Could you check a few things on this model? Use its own coordinates, in mm. A direction names the side the tool comes from. Give positions to 0.01 mm unless a question says otherwise; leave off trailing zeros. Order: outer loops, then holes, each group sorted by start corner. A loop starts at its lowest first (then second) coordinate and runs counter-clockwise, first axis right, second up. Notation, with made-up numbers: M 72,7 L 125,7 A14 ccw 125,33 Z; hole C -34.5,85.25 d10. An arc over 180 degrees is marked long. Return JSON: item names as keys, results as strings. Group by question number.
```python
from build123d import *

# Parameters (mm, degrees)
SKETCH1_R           = 11.25
SKETCH1_R_2         = 1.75
BOSS_EXTRUDE1_DEPTH = 5
BOSS_EXTRUDE2_DEPTH = 46
BOSS_EXTRUDE3_DEPTH = 20
CUT_EXTRUDE1_DEPTH  = 1
CUT_EXTRUDE2_DEPTH  = 65.090268372
CUT_EXTRUDE3_REACH  = 71.748
SKETCH6_R           = 2.7
SKETCH6_R_2         = 3.2
CUT_EXTRUDE4_REACH  = 70.949
SKETCH7_R           = 5.2
SKETCH7_R_2         = 3.2
SKETCH8_R           = 3.05
CUT_EXTRUDE5_DEPTH  = 2
FILLET1_R           = 2.5
FILLET2_R           = 5
FILLET3_R           = 0.5


with BuildPart() as part:
    # Sketch1 → Boss-Extrude1 (new body)
    with BuildSketch(Plane.XY):
        Polygon((-13.5, 34.75), (-28, 20.25), (-28, -7.25), (-0.5, -7.25), (-0.5, -34.75), (7, -34.75), (28, -13.75), (28, 29.75), (23, 34.75), align=None)
        with Locations((7, 13.75)):
            Circle(SKETCH1_R, mode=Mode.SUBTRACT)
        with Locations((-8.5, 29.25)):
            Circle(SKETCH1_R_2, mode=Mode.SUBTRACT)
        with Locations(Location((22.5, 29.25, 0), (0, 0, 180))):
            Circle(SKETCH1_R_2, mode=Mode.SUBTRACT)
        with Locations((22.5, -1.75)):
            Circle(SKETCH1_R_2, mode=Mode.SUBTRACT)
    extrude(amount=BOSS_EXTRUDE1_DEPTH)

    # Sketch2 → Boss-Extrude2 (add)
    with BuildSketch(Plane.XY.offset(5)):
        Polygon((-28, -7.25), (-0.5, -7.25), (-0.5, -34.75), (4.5, -34.75), (4.5, -2.25), (-28, -2.25), align=None)
    extrude(amount=BOSS_EXTRUDE2_DEPTH)

    # Sketch3 → Boss-Extrude3 (add)
    with BuildSketch(Plane(origin=(0, -2.25, 0), x_dir=(1, 0, 0), z_dir=(0, 1, 0))):
        with BuildLine():
            Line((-28, -5), (-28, -17.6))
            Line((-28, -17.6), (-19.6, -26))
            Line((-19.6, -26), (-11.4, -26))
            Line((-11.4, -26), (-4.2, -18.8))
            Line((-4.2, -18.8), (-4.2, -5))
            Line((-4.2, -5), (-18.5, -5))
            Line((-18.5, -5), (-18.5, -11.752647884))
            ThreePointArc((-18.5, -11.752647884), (-11.96959369, -19.81788309), (-19.5, -12.677350455))
            Line((-19.5, -12.677350455), (-19.5, -5))
            Line((-19.5, -5), (-28, -5))
        make_face()
    extrude(amount=BOSS_EXTRUDE3_DEPTH)

    # Sketch4 → Cut-Extrude1 (cut)
    with BuildSketch(Plane(origin=(0, -2.25, 0), x_dir=(1, 0, 0), z_dir=(0, 1, 0))):
        with BuildLine():
            Line((-28, -17.6), (-28, 0))
            Line((-28, 0), (-18.5, 0))
            Line((-18.5, 0), (-18.5, -11.752647884))
            ThreePointArc((-18.5, -11.752647884), (-20.681128714, -15.55738815), (-19.176955262, -19.676955262))
            Line((-19.176955262, -19.676955262), (-22.55, -23.05))
            Line((-22.55, -23.05), (-28, -17.6))
        make_face()
    extrude(amount=CUT_EXTRUDE1_DEPTH, mode=Mode.SUBTRACT)

    # Sketch5 → Cut-Extrude2 (cut, through all)
    with BuildSketch(Plane.XY.offset(5)):
        Polygon((-19.5, 17.75), (-28, 17.75), (-28, 18.75), (-18.5, 18.75), (-18.5, -1.25), (-19.5, -1.25), align=None)
    extrude(amount=-CUT_EXTRUDE2_DEPTH, mode=Mode.SUBTRACT)

    # Sketch6 → Cut-Extrude3 (cut, up to next)
    with BuildSketch(Plane(origin=(4.5, 0, 0), x_dir=(0, 0, -1), z_dir=(1, 0, 0)), mode=Mode.PRIVATE) as cut_extrude3_sk1:
        with Locations((-16, -22.25)):
            Circle(SKETCH6_R)
    cut_extrude3_tool1 = extrude(cut_extrude3_sk1.sketch, amount=-CUT_EXTRUDE3_REACH, mode=Mode.PRIVATE) & part.part
    # Sketch6 → Cut-Extrude3 (cut, up to next)
    with BuildSketch(Plane(origin=(4.5, 0, 0), x_dir=(0, 0, -1), z_dir=(1, 0, 0)), mode=Mode.PRIVATE) as cut_extrude3_sk2:
        with Locations((-37.5, -22.25)):
            Circle(SKETCH6_R_2)
    cut_extrude3_tool2 = extrude(cut_extrude3_sk2.sketch, amount=-CUT_EXTRUDE3_REACH, mode=Mode.PRIVATE) & part.part
    add(cut_extrude3_tool1.solids().sort_by_distance((4.5, -22.25, 16))[0], mode=Mode.SUBTRACT)
    add(cut_extrude3_tool2.solids().sort_by_distance((4.5, -22.25, 37.5))[0], mode=Mode.SUBTRACT)

    # Sketch7 → Cut-Extrude4 (cut, up to next)
    with BuildSketch(Plane(origin=(0, -2.25, 0), x_dir=(1, 0, 0), z_dir=(0, 1, 0)), mode=Mode.PRIVATE) as cut_extrude4_sk1:
        with Locations(Location((-15.5, -16, 0), (0, 0, 125.234417985))):
            Circle(SKETCH7_R)
    cut_extrude4_tool1 = extrude(cut_extrude4_sk1.sketch, amount=-CUT_EXTRUDE4_REACH, mode=Mode.PRIVATE) & part.part
    # Sketch7 → Cut-Extrude4 (cut, up to next)
    with BuildSketch(Plane(origin=(0, -2.25, 0), x_dir=(1, 0, 0), z_dir=(0, 1, 0)), mode=Mode.PRIVATE) as cut_extrude4_sk2:
        with Locations(Location((-15.5, -37.5, 0), (0, 0, 270))):
            Circle(SKETCH7_R_2)
    cut_extrude4_tool2 = extrude(cut_extrude4_sk2.sketch, amount=-CUT_EXTRUDE4_REACH, mode=Mode.PRIVATE) & part.part
    add(cut_extrude4_tool1.solids().sort_by_distance((-15.5, -2.25, 16))[0], mode=Mode.SUBTRACT)
    add(cut_extrude4_tool2.solids().sort_by_distance((-15.5, -2.25, 37.5))[0], mode=Mode.SUBTRACT)

    # Sketch8 → Cut-Extrude5 (cut)
    with BuildSketch(Plane.XY.offset(5)):
        with Locations((-8.5, 29.25)):
            Circle(SKETCH8_R)
    extrude(amount=-CUT_EXTRUDE5_DEPTH, mode=Mode.SUBTRACT)

    # Sketch9 → Cut-Revolve1 (revolve, cut)
    with BuildSketch(Plane(origin=(0, 7.75, 0), x_dir=(1, 0, 0), z_dir=(0, 1, 0)), mode=Mode.PRIVATE) as cut_revolve1_sk:
        Polygon((-4.2, -9), (-4.2, -6), (-7.2, -6), (-7.2, -7.25), (-23, -7.25), (-23, -6.65), (-27, -6.65), (-27, -6.5), (-28, -6.5), (-28, -9), align=None)
    revolve(cut_revolve1_sk.sketch.rotate(Axis((-38.14027768, 7.75, 9), (1, 0, 0)), 180), axis=Axis((-38.14027768, 7.75, 9), (1, 0, 0)), mode=Mode.SUBTRACT)

    # Fillet1
    fillet1_edges = [part.edges().sort_by_distance(p)[0] for p in [
        (4.5, -2.25, 28),
        (-28, 20.25, 2.5),
        (7, -34.75, 2.5),
        (28, -13.75, 2.5),
        (28, 29.75, 2.5),
        (23, 34.75, 2.5),
        (-13.5, 34.75, 2.5),
    ]]
    fillet(fillet1_edges, radius=FILLET1_R)

    # Fillet2
    fillet2_edges = [part.edges().sort_by_distance(p)[0] for p in [
        (-28, 8.25, 17.6),
        (-4.2, 7.75, 18.8),
    ]]
    fillet(fillet2_edges, radius=FILLET2_R)

    # Fillet3
    # the kernel refuses this fillet: 0.5 mm, written as the material it takes off along each edge
    with BuildSketch(Plane(origin=(-28, -1.25, 15.528932188), x_dir=(1, 0, 0), z_dir=(0, 0, -1)), Plane(origin=(-28, 17.75, -1.25), x_dir=(1, 0, 0), z_dir=(0, 0, 1))) as fillet3_piece_1:
        with BuildLine():
            CenterArc((FILLET3_R, -FILLET3_R), FILLET3_R, 90, 90)
            Line((0, -FILLET3_R), (0, 0))
            Line((0, 0), (FILLET3_R, 0))
        make_face()
    extrude(amount=16.778932188, mode=Mode.SUBTRACT)
    with BuildSketch(Plane(origin=(-28, 18.75, 6.272209074), x_dir=(0.0007754462768724465, 0.9999996993414906, 0), z_dir=(0, 0, -1))) as fillet3_piece_2:
        with BuildLine():
            CenterArc((0.500387818, 0.499927816), FILLET3_R, 179.955570197, 91.018024984)
            Line((0.000387968, 0.500315539), (-0.049612017, 0.500354311))
            Line((-0.049612017, 0.500354311), (-0.049999985, 3.8772e-05))
            Line((-0.049999985, 3.8772e-05), (-3.8772e-05, -0.049999985))
            ThreePointArc((-3.8772e-05, -0.049999985), (0.464427182, -0.050360153), (0.509733211, -0.049992782))
            Line((0.509733211, -0.049992782), (0.508883629, 0))
        make_face()
    extrude(amount=7.544418147, mode=Mode.SUBTRACT)
    with BuildSketch(Plane(origin=(-28, -7.25, -1.25), x_dir=(0, 1, 0), z_dir=(0, 0, 1))) as fillet3_piece_3:
        with BuildLine():
            CenterArc((FILLET3_R, -FILLET3_R), FILLET3_R, 90, 90)
            Line((0, -FILLET3_R), (0, 0))
            Line((0, 0), (FILLET3_R, 0))
        make_face()
    extrude(amount=53.5, mode=Mode.SUBTRACT)
    with BuildSketch(Plane(origin=(-26.535533906, 17.75, 19.064466094), x_dir=(0, -1, 0), z_dir=(0.707106781186549, 0, 0.707106781186546))) as fillet3_piece_4:
        with BuildLine():
            CenterArc((FILLET3_R, FILLET3_R), FILLET3_R, 180, 90)
            Line((0, FILLET3_R), (0, 0))
            Line((0, 0), (FILLET3_R, 0))
        make_face()
    extrude(amount=11.058326112, mode=Mode.SUBTRACT)
    with BuildSketch(Plane(origin=(-22.55, -1.25, 23.05), x_dir=(0, 1, 0), z_dir=(-0.7071067811865489, 0, -0.7071067811865461))) as fillet3_piece_5:
        with BuildLine():
            CenterArc((FILLET3_R, FILLET3_R), FILLET3_R, 180, 90)
            Line((0, FILLET3_R), (0, 0))
            Line((0, 0), (FILLET3_R, 0))
        make_face()
    extrude(amount=5.636396103, mode=Mode.SUBTRACT)
    with BuildSketch(Plane(origin=(-23, -1.25, 15.528932188), x_dir=(-0.7071067811865456, 0, 0.7071067811865495), z_dir=(0.7071067811865495, 0, 0.7071067811865456))) as fillet3_piece_6:
        with BuildLine():
            CenterArc((5 - FILLET3_R, -FILLET3_R), FILLET3_R, 0, 90)
            Line((5, -FILLET3_R), (5, 0))
            Line((5, 0), (5 - FILLET3_R, 0))
        make_face()
    revolve(axis=Axis((-23, -1.25, 15.528932188), (0, -1, 0)), revolution_arc=45, mode=Mode.SUBTRACT)
    with BuildSketch(Plane(origin=(-4.2, 17.75, 16.728932188), x_dir=(0, -1, 0), z_dir=(0, 0, -1))) as fillet3_piece_7:
        with BuildLine():
            CenterArc((FILLET3_R, FILLET3_R), FILLET3_R, 180, 90)
            Line((0, FILLET3_R), (0, 0))
            Line((0, 0), (FILLET3_R, 0))
        make_face()
    extrude(amount=11.728932188, mode=Mode.SUBTRACT)
    with BuildSketch(Plane(origin=(-9.2, 17.75, 16.728932188), x_dir=(1, 0, 0), z_dir=(0, 0, -1))) as fillet3_piece_8:
        with BuildLine():
            CenterArc((5 - FILLET3_R, FILLET3_R), FILLET3_R, 270, 90)
            Line((5 - FILLET3_R, 0), (5, 0))
            Line((5, 0), (5, FILLET3_R))
        make_face()
    revolve(axis=Axis((-9.2, 17.75, 16.728932188), (0, -1, 0)), revolution_arc=45, mode=Mode.SUBTRACT)
    with BuildSketch(Plane(origin=(-23, 17.75, 15.528932188), x_dir=(-0.7071067811865456, 0, 0.7071067811865495), z_dir=(0.7071067811865495, 0, 0.7071067811865456))) as fillet3_piece_9:
        with BuildLine():
            CenterArc((5 - FILLET3_R, FILLET3_R), FILLET3_R, 270, 90)
            Line((5, FILLET3_R), (5, 0))
            Line((5, 0), (5 - FILLET3_R, 0))
        make_face()
    revolve(axis=Axis((-23, 17.75, 15.528932188), (0, -1, 0)), revolution_arc=45, mode=Mode.SUBTRACT)
    with BuildSketch(Plane(origin=(-28, -2.25, 52.25), x_dir=(1, 0, 0), z_dir=(0, 0, -1))) as fillet3_piece_10:
        with BuildLine():
            CenterArc((FILLET3_R, FILLET3_R), FILLET3_R, 180, 90)
            Line((0, FILLET3_R), (0, 0))
            Line((0, 0), (FILLET3_R, 0))
        make_face()
    extrude(amount=53.5, mode=Mode.SUBTRACT)
    with BuildSketch(Plane(origin=(-18.5, -2.25, 11.752647884), x_dir=(0, 0, -1), z_dir=(0, 1, 0))) as fillet3_piece_11:
        with BuildLine():
            CenterArc((0.875147274, -0.5), FILLET3_R, 90, 116.014366)
            ThreePointArc((0.425805222, -0.719298246), (0.22737913, -0.351079413), (0, 0))
            Line((0, 0), (0.875147274, 0))
        make_face()
    extrude(amount=22.187868184, mode=Mode.SUBTRACT)
    with BuildSketch(Plane(origin=(-12.283883476, 17.75, 26.883883476), x_dir=(0, -1, 0), z_dir=(0.7071067811865485, 0, -0.7071067811865467))) as fillet3_piece_12:
        with BuildLine():
            CenterArc((FILLET3_R, FILLET3_R), FILLET3_R, 180, 90)
            Line((0, FILLET3_R), (0, 0))
            Line((0, 0), (FILLET3_R, 0))
        make_face()
    extrude(amount=9.361269837, mode=Mode.SUBTRACT)
    with BuildSketch(Plane(origin=(-18.5, 17.75, 5), x_dir=(0, -1, 0), z_dir=(0, 0, 1))) as fillet3_piece_13:
        with BuildLine():
            CenterArc((FILLET3_R, FILLET3_R), FILLET3_R, 180, 90)
            Line((0, FILLET3_R), (0, 0))
            Line((0, 0), (FILLET3_R, 0))
        make_face()
    extrude(amount=8.002647884, mode=Mode.SUBTRACT)
    with BuildSketch(Plane(origin=(-19.5, 17.75, 13.927350455), x_dir=(-1, 0, 0), z_dir=(0, 0, -1))) as fillet3_piece_14:
        with BuildLine():
            CenterArc((FILLET3_R, -FILLET3_R), FILLET3_R, 90, 90)
            Line((0, -FILLET3_R), (0, 0))
            Line((0, 0), (FILLET3_R, 0))
        make_face()
    extrude(amount=15.177350455, mode=Mode.SUBTRACT)
    with BuildSketch(Plane(origin=(-19.5, -1.25, 13.927350455), x_dir=(-1, 0, 0), z_dir=(0, 0, -1))) as fillet3_piece_15:
        with BuildLine():
            CenterArc((FILLET3_R, FILLET3_R), FILLET3_R, 180, 90)
            Line((0, FILLET3_R), (0, 0))
            Line((0, 0), (FILLET3_R, 0))
        make_face()
    extrude(amount=15.177350455, mode=Mode.SUBTRACT)


with BuildPart() as body_2:
    # Mirror1: mirrored copy
    add(part.part.mirror(Plane(origin=(0, 0, 0), x_dir=(0, 0, 1), z_dir=(1, 0, 0))))


solid = body_2.part
```
1. Imagine slicing it at A-A, the plane y = 13.75. Please give me the cut outline in (x, z).
2. Imagine slicing it at B-B, the plane x = 3. Please give me the cut outline in (y, z), plus the area to 3 significant figures.
3. If we mould it in two halves opening along X, with no side actions, what happens to faces 1 (the flat face through (-28, 8, 2)), 2 (the flat face through (-5, 34.75, 2)), 3 (the cylindrical face through (-12.19, 3.77, 2.46))? For each: pulls with the +X half, pulls with the -X half, needs draft (parallel to the pull), parting line crosses it, or undercut.
4. Imagine slicing it at D-D, the plane z = 37. Please give me the cut outline in (x, y).
5. I need wall thicknesses on L1, parallel to Z at x = 13, y = 8.5; L2, parallel to Z at x = -1.5, y = -24.5; L3, parallel to X at y = 29.25, z = 1.55. Which ranges of each line are inside material? Lowest first, please. Write a range as from..to.
6. For pin 1 (2 mm diameter, centred on x = -5, z = 45, fed in from +Y); pin 2 (9 mm diameter, centred on x = 6, z = 21, fed in from +Y); pin 3 (1.5 mm diameter, centred on x = 23.5, z = 2.5, fed in from -Y); pin 4 (5 mm diameter, centred on y = -22.25, z = 16, fed in from -X), each with a flat end and sliding along its axis, tell me the tip position at first contact or that it passes through.
7. Which directions (+Z, -Z, +X, -X, +Y, -Y) give clear straight access to the entire face, cutting with the end or side of a thin tool? Please do faces 4 (the flat face through (23, 8, 11)), 5 (the flat face through (7.2, 8, 11)), 6 (the flat face through (23, 18.75, 3)).
8. Imagine slicing it at C-C, the plane y = -22.25. Please give me the cut outline in (x, z), plus the area to 3 significant figures.
Values:
{
 "1": {"outline": "M -28,0 L -18.25,0 L -18.25,5 L -28,5 Z; M 4.2,5 L 4.25,5 L 4.25,0 L 18.5,0 L 18.5,10.88 A0.5 ccw 17.78,11.33 A5.2 cw long 19.5,12.68 L 19.5,0 L 28,0 L 28,15.53 A5 ccw 26.54,19.06 L 19.6,26 L 11.4,26 L 5.66,20.26 A5 ccw 4.2,16.73 Z"},
 "2": {"outline": "M -7.25,0 L 8.6,0 L 8.6,5 L -2.25,5 L -2.25,51 L -7.25,51 Z; M 18.9,0 L 34.75,0 L 34.75,5 L 18.9,5 Z", "area": "388 mm²"},
 "3": {"face 1": "pulls with the -X half", "face 2": "needs draft", "face 3": "undercut"},
 "4": {"outline": "M -4.5,-34.75 L 0.5,-34.75 L 0.5,-25.41 L -4.5,-25.41 Z; M -4.5,-19.09 L 0.5,-19.09 L 0.5,-7.25 L 12.34,-7.25 L 12.34,-2.25 L -2,-2.25 A2.5 ccw -4.5,-4.75 Z; M 18.66,-7.25 L 27.5,-7.25 A0.5 ccw 28,-6.75 L 28,-2.75 A0.5 ccw 27.5,-2.25 L 18.66,-2.25 Z"},
 "5": {"L1": "z = 0..7.42, 10.58..11.44, 20.56..26", "L2": "z = 0..14.51, 17.49..35.22, 39.78..51", "L3": "x = -27.94..-24.25, -20.75..6.75, 10.25..19"},
 "6": {"pin 1": "stops at y = -3.25", "pin 2": "stops at y = 17.75", "pin 3": "stops at y = -7.25", "pin 4": "passes through"},
 "7": {"face 4": "+X", "face 5": "-X", "face 6": "+Z, -Z, +X"},
 "8": {"outline": "M -19.5,0 L 0.5,0 L 0.5,13.3 L -4.5,13.3 L -4.5,5 L -19.5,5 Z; M -4.5,18.7 L 0.5,18.7 L 0.5,34.3 L -4.5,34.3 Z; M -4.5,40.7 L 0.5,40.7 L 0.5,51 L -4.5,51 Z", "area": "271 mm²"}
}
